Input: part model. Units: mm. Frame: model coordinates. Round coordinates to 2 decimals unless told otherwise and drop trailing zeros. Loops run counter-clockwise (first coordinate to the right, second up) from the corner with the lowest first, then second, coordinate; pieces in that order, holes last. Notation, with made-up numbers: M -23,45 L 0,45 A19 ccw 0,55 Z; hole C 25,30 d3. An arc over 180 degrees is marked long. Return JSON: item names as keys, results as strings. Group by question number.
1) Section A-A (x = 80). Output: boundary loops of the cut face in (y, z), plus the area to 3 significant figures.
2) Contact query for flat-ended pins moving along their axis: P1, Ø1.4, axis at x = 63, y = -4, coming from the -Z side; P2, Ø4, axis at x = 57, y = -5, coming from the -Z side. Output: stop coordinate, or through.
3) Material intervals for line 1 (Y direction, x = 8, z = 1.25); line 2 (Z direction, x = 27, y = -3.25); line 3 (Z direction, x = 62.5, y = -2.5), sorted ascending. Write a range as from..to.
from build123d import *

# Parameters (mm, degrees)
F1_DEPTH  = 8
F3_W      = 8
F3_H      = 8
F3_R      = 2.4
F4_DEPTH  = 1.7
F5_R      = 2.4
F6_DEPTH  = 1.7
F14_W     = 31.3753262162
F14_H     = 26.4205296278
F15_DEPTH = 32.004


with BuildPart() as f1:
    # F0 (on Front) → F1 (new body)
    with BuildSketch(Plane.XZ):
        Polygon((-2.4, 3.2), (-4, 3.2), (-4, 0), (4, 0), (4, 3.2), (2.4, 3.2), (2.4, 4.9), (-2.4, 4.9), align=None)
    extrude(amount=F1_DEPTH)

    # F3 (on plane+point) → F4 (cut, through all)
    with BuildSketch(Plane.XY.offset(4.9)):
        with Locations((0, -4)):
            Rectangle(F3_W, F3_H)
        with Locations((0, -4)):
            Circle(F3_R, mode=Mode.SUBTRACT)
    extrude(amount=-F4_DEPTH, mode=Mode.SUBTRACT)

    # F5 (on Top) → F6 (cut)
    with BuildSketch(Plane.XY):
        with Locations((0, -4)):
            Circle(F5_R)
    extrude(amount=F6_DEPTH, mode=Mode.SUBTRACT)

    # F8: F1 across plane


with BuildPart() as f1_1:
    add(f1.part)
    add(f1.part.mirror(Plane.YZ.offset(4)))

    # F10: F1 across plane


with BuildPart() as f1_2:
    add(f1_1.part)
    add(f1_1.part.mirror(Plane.YZ.offset(12)))

    # F12: F1 across plane


with BuildPart() as f1_3:
    add(f1_2.part)
    add(f1_2.part.mirror(Plane.YZ.offset(28)))

    # F13: F1 across face


with BuildPart() as f1_4:
    add(f1_3.part)
    add(f1_3.part.mirror(Plane(origin=(60, -4, 1.6), x_dir=(0, 1, 0), z_dir=(1, 0, 0))))

    # F14 (on face) → F15 (cut)
    with BuildSketch(Plane.YZ.offset(124)):
        with Locations((0, 3.2)):
            Rectangle(F14_W, F14_H)
    extrude(amount=-F15_DEPTH, mode=Mode.SUBTRACT)


solid = f1_4.part
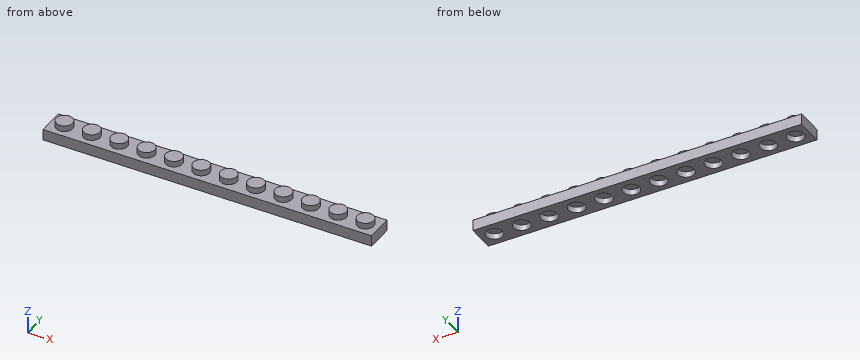
Returned:
{
 "1": {"outline": "M -8,0 L -6.4,0 L -6.4,1.7 L -1.6,1.7 L -1.6,0 L 0,0 L 0,3.2 L -1.6,3.2 L -1.6,4.9 L -6.4,4.9 L -6.4,3.2 L -8,3.2 Z", "area": "25.6 mm^2"},
 "2": {"P1": "stops at z = 1.7", "P2": "stops at z = 0"},
 "3": {"line 1": "y = -8..-6.4, -1.6..0", "line 2": "z = 0..3.2", "line 3": "z = 1.7..4.9"}
}
